The model under review builds one solid part; all positions refer to its coordinate system, in mm. A direction names the side the tool comes from. Coordinates: 2 decimals unless noted, no trailing zeros. Loops run counter-clockwise (first coordinate to the right, second up) from the corner with the lowest first, then second, coordinate; pieces in that order, holes last. Notation, with made-up numbers: M 39.5,-33 L 77.5,-33 A28 ccw 77.5,-5 Z; hole C 0,-0.75 d5. An arc over 180 degrees is marked long. Write item = value, one per line. Start each with the question number.
Q1. We need section C-C on z = -221. Give the boundary of the cut face in (x, y) (3 decimals).
Q2. We need section B-B on y = 342.5. Give the boundary of the cut face in (x, z) (3 decimals), and give its area (3 significant figures).
Q3. Clearance check with flat-ended pins moving along their axes: pin 1 Ø8 at (x, z) = (7, -172.5) entering from +Y; pin 2 Ø6 at (x, y) = (11.5, 445.5) entering from -Z; pin 3 Ø4 at (x, y) = (15.5, 171.5) entering from -Z. State where each tip first meets the part, or that it passes through.
Q4. Wall thickness on probe 1 along Z at (x, y) = (9, 347) (3 decimals); probe 2 along Y at (x, z) = (12.25, -354.5) (3 decimals); probe 3 along Y at (x, z) = (3, -177) (3 decimals): over which ranges is each line inside the solid? List them lowest first.
Q5. For faces 1 (the face through (18.256, 239, -239)), 2 (the face through (9.256, 176.512, -382.887)), list the 3-axis set-ups (+Z, -Z, +X, -X, +Y, -Y) from which the entire face can be reached by the end or side of a thin tool; tool diameter is ignored.
Q6. We need section D-D on y = 497. Give the boundary of the cut face in (x, z), and give its area (3 significant figures).
from build123d import *

# Parameters (mm, degrees)
BOSS_EXTRUDE1_DEPTH = 18.25625
CUT_EXTRUDE2_DEPTH  = 854.319644485
FILLET2_R           = 3.3782


with BuildPart() as part:
    # Sketch1 → Boss-Extrude1 (new body)
    with BuildSketch(Plane(origin=(0, 0, 0), x_dir=(0, 0, -1), z_dir=(1, 0, 0))):
        Polygon((0, 0), (0, 603.25), (88.9, 603.25), (603.25, 88.9), (603.25, 0), align=None)
    extrude(amount=BOSS_EXTRUDE1_DEPTH)

    # Sketch7 → Cut-Extrude2 (cut, through all)
    with BuildSketch(Plane(origin=(18.25625, 0, 0), x_dir=(0, 0, -1), z_dir=(1, 0, 0))):
        Polygon((200.025, 406.4), (406.4, 200.025), (358.775, 152.4), (152.4, 358.775), align=None)
    extrude(amount=-CUT_EXTRUDE2_DEPTH, mode=Mode.SUBTRACT)

    # Fillet2
    fillet2_edges = [part.edges().sort_by_distance(p)[0] for p in [
        (9.128125, 358.775, -152.4),
        (9.128125, 406.4, -200.025),
        (9.128125, 200.025, -406.4),
        (9.128125, 152.4, -358.775),
    ]]
    fillet(fillet2_edges, radius=FILLET2_R)


solid = part.part
Returned:
q1.outline = M 0,0 L 18.256,0 L 18.256,290.175 L 0,290.175 Z; M 0,385.425 L 18.256,385.425 L 18.256,471.15 L 0,471.15 Z
q2.outline = M 0,-349.65 L 18.256,-349.65 L 18.256,-263.925 L 0,-263.925 Z; M 0,-168.675 L 18.256,-168.675 L 18.256,0 L 0,0 Z
q2.area = 4,640 mm^2
q3.pin_1 = 523.65
q3.pin_2 = -249.65
q3.pin_3 = -522.65
q4.probe_1 = -345.15 to -259.425, -164.175 to 0
q4.probe_2 = 0 to 156.675, 251.925 to 337.65
q4.probe_3 = 0 to 334.175, 383.375 to 515.15
q5.face_1 = +Z, -Z, +X, +Y, -Y
q5.face_2 = +X, -X
q6.outline = M 0,-195.15 L 18.26,-195.15 L 18.26,0 L 0,0 Z
q6.area = 3,560 mm^2
